Part model, mm, in its own coordinate system. Round coordinates to 2 decimals unless told otherwise and drop trailing zeros. Order: outer loops, then holes, each group sorted by start corner. A loop starts at its lowest first (then second) coordinate and runs counter-clockwise, first axis right, second up. Notation, with made-up numbers: M -7,16.25 L 35,16.25 A28 cw 35,43.25 Z; hole C 79,-18.75 d3. An arc over 180 degrees is marked long. One line per question, with ' | ' between items.
from build123d import *

# Parameters (mm, degrees)
SKETCH3_R           = 3.5
BOSS_EXTRUDE1_DEPTH = 2.5


with BuildPart() as part:
    # Sketch3 → Boss-Extrude1 (new body)
    with BuildSketch(Plane(origin=(0, 0, 0), x_dir=(1, 0, 0), z_dir=(0, 1, 0))):
        Polygon((-9.459826986, 67.208739943), (9.459826986, 67.208739943), (13.231926916, 70.980839873), (17.154910843, 70.980839873), (24.321900711, 63.813850005), (24.321900711, 31.751000599), (20.738405777, 28.167505665), (29.829166609, 16.360832883), (29.829166609, -16.360832883), (20.738405777, -28.167505665), (24.321900711, -31.751000599), (24.321900711, -63.813850005), (17.154910843, -70.980839873), (13.231926916, -70.980839873), (9.459826986, -67.208739943), (-9.459826986, -67.208739943), (-13.231926916, -70.980839873), (-17.154910843, -70.980839873), (-24.321900711, -63.813850005), (-24.321900711, -31.751000599), (-20.738405777, -28.167505665), (-29.829166609, -16.360832883), (-29.829166609, 16.360832883), (-20.738405777, 28.167505665), (-24.321900711, 31.751000599), (-24.321900711, 63.813850005), (-17.154910843, 70.980839873), (-13.231926916, 70.980839873), align=None)
        with Locations(Location((23.5, 0, 0), (0, 0, 270))):
            Circle(SKETCH3_R, mode=Mode.SUBTRACT)
        with Locations(Location((-23.5, 0, 0), (0, 0, 90))):
            Circle(SKETCH3_R, mode=Mode.SUBTRACT)
        with Locations(Location((0, 50, 0), (0, 0, 270))):
            Circle(SKETCH3_R, mode=Mode.SUBTRACT)
        with Locations(Location((0, -50, 0), (0, 0, 90))):
            Circle(SKETCH3_R, mode=Mode.SUBTRACT)
        Polygon((-2.79989697, 38.028097822), (2.79989697, 38.028097822), (3.941780629, 40.002717551), (7.169853306, 40.002717551), (8.795336711, 38.028097822), (8.795336711, 31.028097822), (7.169853306, 29.053478092), (3.941780629, 29.053478092), (2.79989697, 31.028097822), (-2.79989697, 31.028097822), (-3.941780629, 29.053478092), (-7.169853306, 29.053478092), (-8.795336711, 31.028097822), (-8.795336711, 38.028097822), (-7.169853306, 40.002717551), (-3.941780629, 40.002717551), align=None, mode=Mode.SUBTRACT)
        Polygon((-2.79989697, -31.028097822), (-3.941780629, -29.053478092), (-7.169853306, -29.053478092), (-8.795336711, -31.028097822), (-8.795336711, -38.028097822), (-7.169853306, -40.002717551), (-3.941780629, -40.002717551), (-2.79989697, -38.028097822), (2.79989697, -38.028097822), (3.941780629, -40.002717551), (7.169853306, -40.002717551), (8.795336711, -38.028097822), (8.795336711, -31.028097822), (7.169853306, -29.053478092), (3.941780629, -29.053478092), (2.79989697, -31.028097822), align=None, mode=Mode.SUBTRACT)
    extrude(amount=BOSS_EXTRUDE1_DEPTH)


solid = part.part
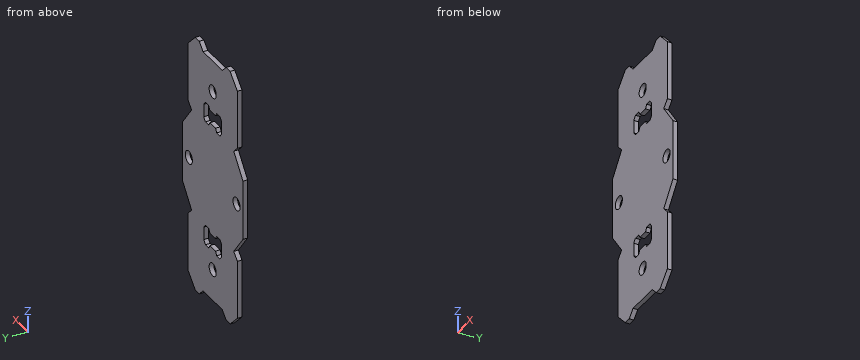
1) Saw through at D-D (y = 1.1). Give the number of separate pieces and of enclosed holes in the cut face, plus the area to 3 significant figures.
The answers:
separate pieces: 1 | enclosed holes: 6 | area: 6,540 mm²
2) Probe line 1 (X direction, y = 1.9, z = 0); line 2 (X direction, y = 1.65, z = 50); line 3 (Z direction, x = -7.5, y = 2.25). List the from-to ranges inside material, lowest first. Write a range as [from, to].
The answers:
line 1: x = [-29.83, -27], [-20, 20], [27, 29.83] | line 2: x = [-24.32, -3.5], [3.5, 24.32] | line 3: z = [-67.21, -39.6], [-29.45, 29.45], [39.6, 67.21]
3) Saw through at B-B (z = -50). List the corners of the cut face in (x, y), plus the area to 3 significant figures.
The answers:
outline: M -24.32,0 L -3.5,0 L -3.5,2.5 L -24.32,2.5 Z; M 3.5,0 L 24.32,0 L 24.32,2.5 L 3.5,2.5 Z | area: 104 mm²
4) Saw through at C-C (z = 0). List the corners of the cut face in (x, y), plus the area to 3 significant figures.
The answers:
outline: M -29.83,0 L -27,0 L -27,2.5 L -29.83,2.5 Z; M -20,0 L 20,0 L 20,2.5 L -20,2.5 Z; M 27,0 L 29.83,0 L 29.83,2.5 L 27,2.5 Z | area: 114 mm²
5) Saw through at A-A (x = 0). List the corners of the cut face in (y, z).
The answers:
outline: M 0,-67.21 L 2.5,-67.21 L 2.5,-53.5 L 0,-53.5 Z; M 0,-46.5 L 2.5,-46.5 L 2.5,-38.03 L 0,-38.03 Z; M 0,-31.03 L 2.5,-31.03 L 2.5,31.03 L 0,31.03 Z; M 0,38.03 L 2.5,38.03 L 2.5,46.5 L 0,46.5 Z; M 0,53.5 L 2.5,53.5 L 2.5,67.21 L 0,67.21 Z
6) Drop flat-ended pins along their axis: pin 1 (0.8 mm diameter, centred on y = 1, z = -33, fed in from -X); pin 2 (1.2 mm diameter, centred on x = -5.5, y = 1, fed in from +Z); pin 3 (0.8 mm diameter, centred on y = 1, z = -33.5, fed in from +X); pin 4 (4 mm diameter, centred on x = 0, z = -50, fed in from +Y). Give the stop position or say it passes through.
The answers:
pin 1: stops at x = -24.32 | pin 2: stops at z = 67.21 | pin 3: stops at x = 24.32 | pin 4: passes through
